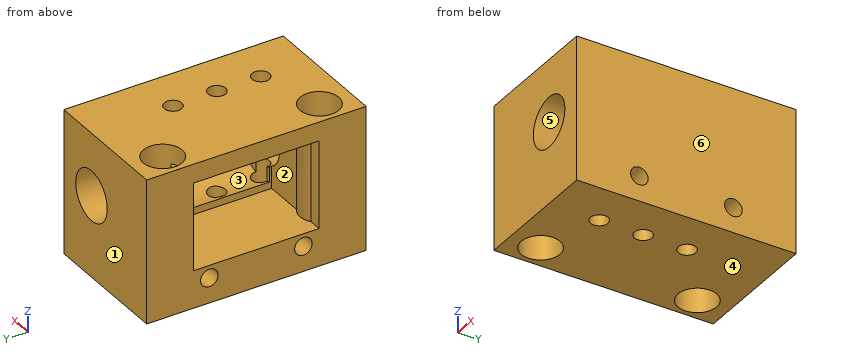
Autodesk Inventor part; units mm, degrees
ref_plane "Work Plane2" through (-3.5, -134.0004, -5) normal (0, 0, -1) x (0, 1, 0)
ref_plane "YZ Plane" through (0, 0, 0) normal (1, 0, 0) x (0, 1, 0)
ref_plane "XZ Plane" through (0, 0, 0) normal (0, 1, 0) x (-1, 0, 0)
sketch "Sketch1" plane through (0, 0, 0) normal (1, 0, 0) x (0, 1, 0)
  line L0 (0, 0) -> (35, 0)
  line L1 (35, 0) -> (35, 20)
  line L2 (35, 20) -> (0, 20)
  line L3 (0, 20) -> (0, 0)
  dimension "d0" = 35
  dimension "d1" = 20
extrude "Extrusion1" add sketch "Sketch1" along normal blind 14
ref_plane "Work Plane1" through (7, 0, 0) normal (-1, 0, 0) x (0, 0, 1)
sketch "Sketch2" plane through (7, 0, 0) normal (-1, 0, 0) x (0, 0, 1)
  line L0 (20, 0) -> (0, 0)
  line L1 (10, 0) -> (10, 35)
  line L2 (0, 35) -> (20, 35)
  line L3 (3.8, 7.9) -> (16.2, 7.9)
  line L4 (16.2, 7.9) -> (16.2, 27.1)
  line L5 (16.2, 27.1) -> (3.8, 27.1)
  line L6 (3.8, 27.1) -> (3.8, 7.9)
  line L7 (3.8, 7.9) -> (16.2, 27.1) construction
  line L8 (16.2, 7.9) -> (3.8, 27.1) construction
  line L9 (10, 7.9) -> (6, 7.9)
  line L10 (6, 7.9) -> (6, 0)
  line L11 (6, 0) -> (10, 0)
  line L12 (10, 0) -> (10, 7.9)
  line L13 (10, 27.1) -> (6, 27.1)
  line L14 (6, 27.1) -> (6, 35)
  line L15 (6, 35) -> (10, 35)
  line L16 (10, 35) -> (10, 27.1)
  line L17 (10, 27.1) -> (3.8, 27.1)
  line L18 (3.8, 27.1) -> (3.8, 7.9)
  line L19 (3.8, 7.9) -> (10, 7.9)
  line L20 (10, 7.9) -> (10, 27.1)
  point P0 (10, 17.5)
  dimension "d5" = 12.4
  dimension "d6" = 19.2
  dimension "d7" = 4
revolve "Revolution1" cut sketch "Sketch2" angle 360 about axis through (7, 0, 10) along (0, 1, 0) contours L0 L10 L3 L1 | L3 L6 L5 L1 | L5 L14 L2 L1
sketch "Sketch3" plane through (0, 0, 20) normal (0, 0, 1) x (1, 0, 0)
  line L0 (0, 35) -> (0, 0)
  line L1 (0, 0) -> (14, 0)
  line L2 (14, 35) -> (14, 0)
  line L3 (0, 35) -> (14, 35)
  line L4 (0, 0) -> (0, 35)
  line L5 (0, 0) -> (-7, 0)
  line L6 (-7, 0) -> (-7, 35)
  line L7 (-7, 35) -> (0, 35)
  line L8 (0, 35) -> (0, 0)
  line L9 (0, 35) -> (14, 35)
  circle A0 centre (-3.1, 5) radius 3.1
  line L10 (0, 35) -> (0, 0)
  circle A1 centre (-3.1, 30) radius 3.1
  dimension "d9" = 7
  dimension "d10" = 6.2
  dimension "d11" = 6.2
  dimension "d12" = 5
  dimension "d13" = 5
extrude "Extrusion2" add sketch "Sketch3" against normal up to surface (20 mm away) contours L0 L5 L6 L7
sketch "Sketch4" plane through (-7, 0, 20) normal (-1, 0, 0) x (0, 0, 1)
  line L0 (-16.2, 27.1) -> (-16.2, 7.9)
  line L1 (-15, 24.5) -> (-5, 24.5)
  line L2 (-14, 27.1) -> (-6, 27.1)
  line L3 (-16.2, 7.9) -> (-3.8, 7.9)
  line L4 (-3.8, 27.1) -> (-3.8, 7.9)
  line L5 (-16.2, 27.1) -> (-3.8, 27.1)
  line L6 (-17, 27.5113) -> (-3, 27.5113)
  line L7 (-3, 27.5113) -> (-3, 7.5113)
  line L8 (-3, 7.5113) -> (-17, 7.5113)
  line L9 (-17, 7.5113) -> (-17, 27.5113)
  line L10 (-17, 27.5113) -> (-3, 7.5113) construction
  line L11 (-3, 27.5113) -> (-17, 7.5113) construction
  line L12 (-13.5, 32.7798) -> (-6.5, 32.7798)
  line L13 (-6.5, 32.7798) -> (-6.5, 27.5113)
  line L14 (-6.5, 27.5113) -> (-13.5, 27.5113)
  line L15 (-13.5, 27.5113) -> (-13.5, 32.7798)
  line L16 (-13.5, 32.7798) -> (-6.5, 27.5113) construction
  line L17 (-6.5, 32.7798) -> (-13.5, 27.5113) construction
  line L18 (-13.5, 1.8013) -> (-6.5, 1.8013)
  line L19 (-6.5, 1.8013) -> (-6.5, 7.5113)
  line L20 (-6.5, 7.5113) -> (-13.5, 7.5113)
  line L21 (-13.5, 7.5113) -> (-13.5, 1.8013)
  line L22 (-13.5, 1.8013) -> (-6.5, 7.5113) construction
  line L23 (-6.5, 1.8013) -> (-13.5, 7.5113) construction
  line L24 (0, 35) -> (-20, 35)
  line L25 (-13.5, 32.7798) -> (-6.5, 32.7798)
  line L26 (-6.5, 32.7798) -> (-6.5, 35)
  line L27 (-6.5, 35) -> (-13.5, 35)
  line L28 (-13.5, 35) -> (-13.5, 32.7798)
  line L29 (-6, 0) -> (-14, 0)
  line L30 (-13.5, 1.8013) -> (-6, 1.8013)
  line L31 (-6, 1.8013) -> (-6, 0)
  line L32 (-6, 0) -> (-13.5, 0)
  line L33 (-13.5, 0) -> (-13.5, 1.8013)
  point P0 (-20, 0)
  point P1 (-10, 17.5113)
  point P2 (-10, 30.1456)
  point P3 (-10, 4.6563)
  dimension "d16" = 14
  dimension "d17" = 20
  dimension "d18" = 7
  dimension "d41" = 7
extrude "Extrusion3" cut sketch "Sketch4" against normal blind 12 contours L5 L2 L4 L3 L0 | L6 L7 L8 L9
sketch "Sketch5" plane through (14, 0, 0) normal (0, 0, -1) x (-1, 0, 0)
  line L0 (21, 35) -> (0, 35)
  line L1 (0, 0) -> (0, 35)
  line L2 (21, 0) -> (0, 0)
  line L3 (21, 35) -> (21, 0)
  circle A0 centre (17.1, 30) radius 3.1
  circle A1 centre (17.1, 5) radius 3.1
  point P0 (14, 0)
ref_plane "Work Plane2" through (-3.5, -134.0004, -5) normal (0, 0, -1) x (0, 1, 0)
extrude "Extrusion4" add sketch "Sketch5" along normal blind 3
sketch "Sketch6" plane through (-7, 0, 20) normal (-1, 0, 0) x (0, 0, 1)
  point P0 (-20, 0)
sketch "Sketch7" plane through (-7, 0, 20) normal (-1, 0, 0) x (0, 0, 1)
  line L0 (-3, 7.5113) -> (-17, 7.5113)
  line L1 (-17, 7.5113) -> (-17, 27.5113)
  line L2 (-17, 27.5113) -> (-3, 27.5113)
  line L3 (-3, 27.5113) -> (-3, 7.5113)
  line L4 (0, 0) -> (-23, 0)
  line L5 (0, 35) -> (0, 0)
  line L6 (0, 35) -> (-23, 35)
  line L7 (-23, 0) -> (-23, 35)
  circle A0 centre (-19, 10) radius 1.4
  circle A1 centre (-19, 25) radius 1.4
  point P0 (-20, 0)
  dimension "d23" = 2.8
  dimension "d24" = 2.8
  dimension "d25" = 10
  dimension "d26" = 10
  dimension "d27" = 4
  dimension "d36" = 4
extrude "Extrusion5" cut sketch "Sketch7" against normal through all contours A0 | A1
sketch "Sketch8" plane through (14, 0, 20) normal (0, 0, 1) x (1, 0, 0)
  line L0 (-10, 99.8613) -> (-10, -100.1387)
  line L1 (-4, 99.8613) -> (-4, -100.1387)
  circle A0 centre (-7, 15) radius 1.4
  line L2 (-21, 0) -> (0, 0)
  circle A1 centre (-7, 8) radius 1.4
  circle A2 centre (-7, 22) radius 1.4
  point P0 (-14, 0)
  dimension "d31" = 2.8
  dimension "d32" = 15
  dimension "d33" = 3
  dimension "d37" = 2.8
  dimension "d38" = 2.8
  dimension "d39" = 7
  dimension "d40" = 7
extrude "Extrusion6" cut sketch "Sketch8" against normal through all
properties part number "30_CUBE_openXY_slider"
Source: CAD feature listing. Evaluate the final solid. Frame: model axes, mm. Face numbers are marked on the shaded views. A direction names the side the tool comes from. Round coordinates to 2 decimals unless told otherwise and drop trailing zeros. Loops run counter-clockwise (first coordinate to the right, second up) from the corner with the lowest first, then second, coordinate; pieces in that order, holes last.
1. Section query B-B on z = 1. Output: boundary loops of the cut face in (x, y).
2. Contact query for flat-ended pins moving along their axis: pin 1 (1.5 mm diameter, centred on y = 10, z = 10, fed in from -X); pin 2 (1.1 mm diameter, centred on y = 15.5, z = 5, fed in from -X). Output: stop coordinate, or through.
3. Ray query, L1, parallel to Y at x = 7, z = 18.4; L2, parallel to Y at x = 5.5, z = 1; L3, parallel to Y at x = 7, z = 15.75. Return the intervals inside material, ascending.
4. Mould query, pull axis Z, two halves, no side actions, for the marked faces 4, 5 and 6. Classes: released by +Z, released by -Z, zero draft, split by the parting line, or undercut.
5. Access query for the marked faces 1, 2 and 3. Directions: +Z, -Z, +X, -X, +Y, -Y. A direction counts if a zero-diameter tool reaches every point of the face in a straight line with its end or side. Return the directions, or none.
6. Section query D-D on y = 25. Output: boundary loops of the cut face in (x, z).
7. Section query A-A on y = 5. Output: boundary loops of the cut face in (x, z), and give its area (3 significant figures).
8. Section query C-C on x = 4.5. Output: boundary loops of the cut face in (y, z), and give its area (3 significant figures).
Answers below:
1. outline: (-7, 0) - (14, 0) - (14, 8.6) - (8.26, 8.6) arc R1.4 cw (long way) to (5.74, 8.6) - (-7, 8.6) - close; (-7, 11.4) - (14, 11.4) - (14, 23.6) - (-7, 23.6) - close; (-7, 26.4) - (14, 26.4) - (14, 35) - (-7, 35) - close; hole circle Ø6.2 at (-3.1, 5); hole circle Ø6.2 at (-3.1, 30); hole circle Ø2.8 at (7, 15); hole circle Ø2.8 at (7, 22)
2. pin 1: stops at x = 13.15
2. pin 2: stops at x = 9.76
3. L1: y = 0 to 6.6, 9.4 to 13.6, 16.4 to 20.6, 23.4 to 35
3. L2: y = 0 to 8.6, 11.4 to 23.6, 26.4 to 35
3. L3: y = 0 to 6.6, 27.1 to 35
4. face 4: released by -Z
4. face 5: undercut
4. face 6: zero draft
5. face 1: +Z, -Z, +X, -X, +Y
5. face 2: -X
5. face 3: none
6. outline: (-7, -3) - (14, -3) - (14, -0.4) - (-7, -0.4) - close; (-7, 2.4) - (14, 2.4) - (14, 20) - (-7, 20) - (-7, 17) - (5, 17) - (5, 15.87) arc R6.2 cw (long way) to (5, 4.13) - (5, 3) - (-7, 3) - close
7. outline: (-7, -3) - (-6.2, -3) - (-6.2, 20) - (-7, 20) - close; (0, -3) - (14, -3) - (14, 20) - (0, 20) - close; hole circle Ø8 at (7, 10)
7. area: 290 mm2
8. outline: (0, -3) - (35, -3) - (35, 6.88) - (27.51, 6.88) - (27.51, 3) - (7.51, 3) - (7.51, 6.88) - (0, 6.88) - close; (0, 13.12) - (7.51, 13.12) - (7.51, 17) - (27.51, 17) - (27.51, 13.12) - (35, 13.12) - (35, 20) - (0, 20) - close; hole circle Ø2.8 at (10, 1); hole circle Ø2.8 at (25, 1)
8. area: 419 mm2
